from build123d import *

# Parameters (mm, degrees)
ZAOKR_GLENIE1_R             = 1
SFAZOWANIE1_SIZE            = 0.3
SFAZOWANIE1_SIZE2           = 1.701384546
SZKIC2_W                    = 0.5
SZKIC2_H                    = 2
DODANIE_WYCI_GNI_CIE1_DEPTH = 5


with BuildPart() as part:
    # Szkic1 → Obrót1 (revolve)
    with BuildSketch(Plane(origin=(0, 0, 0), x_dir=(0, 0, -1), z_dir=(1, 0, 0))):
        Polygon((2, 0), (12, 0), (12, 3.5), (11, 3.5), (11, 4), (4, 4), (4, 5), (0, 5), (0, 2.5), (8, 2.5), (8, 1.1), (2, 1.1), align=None)
    revolve(axis=Axis((0, 0, 23.697784827), (0, 0, -1)))

    # Zaokrąglenie1
    zaokr_glenie1_edges = [part.edges().sort_by_distance(p)[0] for p in [
        (0, -1.1, -2),
    ]]
    fillet(zaokr_glenie1_edges, radius=ZAOKR_GLENIE1_R)

    # Sfazowanie1
    sfazowanie1_edges = [part.edges().sort_by_distance(p)[0] for p in [
        (0, -2.5, 0),
    ]]
    sfazowanie1_side = [part.faces().sort_by_distance(p)[0] for p in [
        (0, -2.5, -4),
    ]]
    chamfer(sfazowanie1_edges, length=SFAZOWANIE1_SIZE, length2=SFAZOWANIE1_SIZE2, reference=sfazowanie1_side[0])

    # Szkic2 → Dodanie-wyciągnięcie1 (add)
    with BuildSketch(Plane(origin=(0, 0, -12), x_dir=(-1, 0, 0), z_dir=(0, 0, -1))):
        with Locations((-2.5, 0)):
            Rectangle(SZKIC2_W, SZKIC2_H)
        Rectangle(SZKIC2_W, SZKIC2_H)
    extrude(amount=DODANIE_WYCI_GNI_CIE1_DEPTH)


solid = part.part
Design review of the part built by this model. Coordinates are the model's own, in mm. A direction names the side the tool comes from. Give positions to 0.01 mm unless a question says otherwise; leave off trailing zeros. Loops run counter-clockwise (first coordinate to the right, second up) from the corner with the lowest first, then second, coordinate; pieces in that order, holes last. Notation, with made-up numbers: M 84.5,8.25 L 94.5,8.25 A24 ccw 94.5,20.25 Z; hole C 44.25,89 d4. An arc over 180 degrees is marked long. Answer as a JSON object with one key per item and string values.
Item 1: We need section A-A (z = -13.75). State the section outline as (x, y) points.
Output values:
{"outline": "M -0.25,-1 L 0.25,-1 L 0.25,1 L -0.25,1 Z; M 2.25,-1 L 2.75,-1 L 2.75,1 L 2.25,1 Z"}
Item 2: Wall thickness on line 1 along X through (y, z) = (0, -5.5); line 2 along X through (y, z) = (0, -3); line 3 along Y through (x, z) = (-0.5, -6.25): over which ranges is each line inside the solid? List them lowest first.
Output values:
{"line 1": "x = -4 to -2.5, -1.1 to 1.1, 2.5 to 4", "line 2": "x = -5 to -2.5, -1.1 to 1.1, 2.5 to 5", "line 3": "y = -3.97 to -2.45, -0.98 to 0.98, 2.45 to 3.97"}
Item 3: We need section C-C (z = -10.75). State the section outline as (x, y) points.
Output values:
{"outline": "C 0,0 d8"}
Item 4: Mouldability with a two-part tool opening along X and no side actions: class faces 4 (the face through (2.75, 0, -14)), 5 (the face through (0.25, 0, -14)), 6 (the face through (-4.88, -1.08, -1.97)) as pulls with the +X half, pulls with the -X half, needs draft (parallel to the pull), parting line crosses it, or undercut.
Output values:
{"face 4": "pulls with the +X half", "face 5": "undercut", "face 6": "parting line crosses it"}
Item 5: We need section D-D (z = -2.25). Count the separate pieces of the cut face and the enclosed holes in it, and give its area (3 significant figures).
Output values:
{"separate pieces": "2", "enclosed holes": "1", "area": "60.7 mm2"}
Item 6: For P1, Ø2, axis at y = 0, z = -15, coming from the -X side; P2, Ø6, axis at x = -3.5, z = -2, coming from the -Y side; P3, Ø2, axis at y = -0.5, z = -15, coming from the +X side, all flat-tipped, find the tip position at first contact; note any pin that passes through.
Output values:
{"P1": "stops at x = -0.25", "P2": "stops at y = -4.97", "P3": "stops at x = 2.75"}
Item 7: Machinability: for faces 1 (the face through (-1.341, 3.233, -11.493)), 2 (the face through (-0.25, 0, -14)), 3 (the face through (-1, 1, -8)), which of the approach directions +Z, -Z, +X, -X, +Y, -Y give a long, thin tool a straight path to every point of the face, cutting with its end or side? Answer none if there is none.
Output values:
{"face 1": "-Z", "face 2": "-Z, -X, +Y, -Y", "face 3": "+Z"}
Item 8: We need section B-B (z = -7.5). State the section outline as (x, y) points.
Output values:
{"outline": "C 0,0 d8; C 0,0 d2.2; hole C 0,0 d5"}
